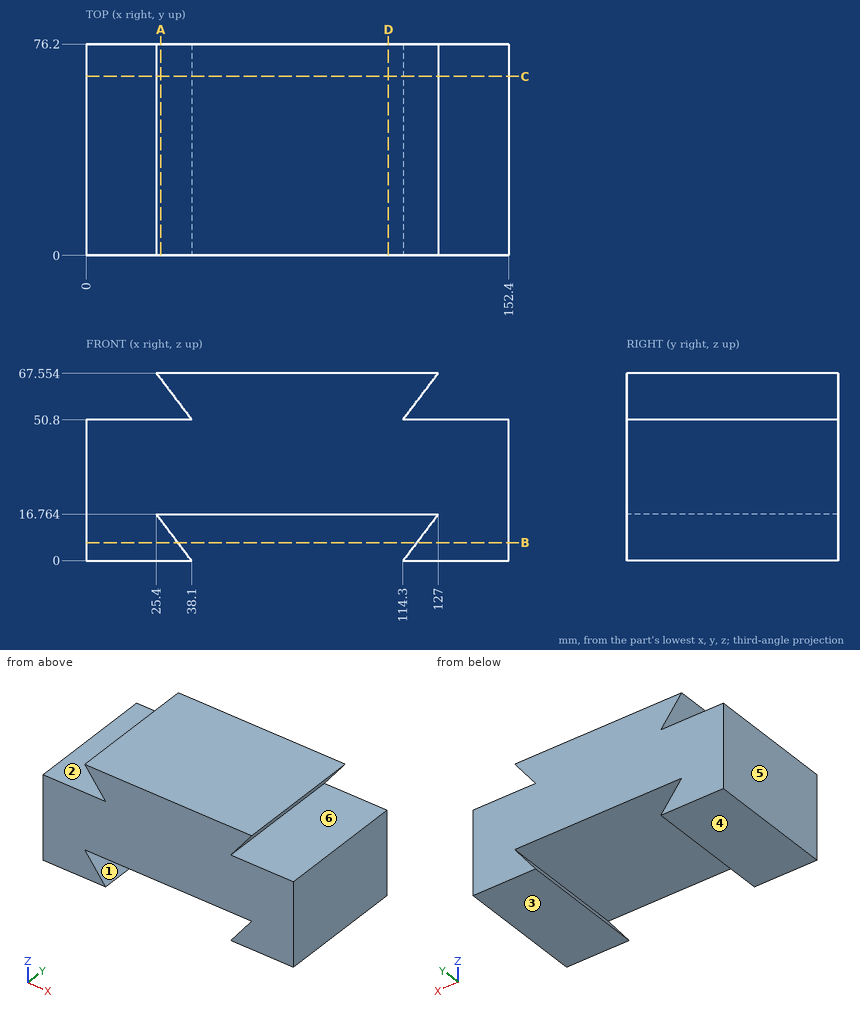
Here's the drawing with two shaded views (mm, measured from the low corner). I have some questions. A direction names the side the tool comes from. Give positions to 0.01 mm unless a question says otherwise; leave off trailing zeros. Order: outer loops, then holes, each group sorted by start corner. A loop starts at its lowest first (then second) coordinate and runs counter-clockwise, first axis right, second up. Notation, with made-up numbers: M 11.5,41 L 47.5,41 A16 cw 47.5,60 Z; hole C 5,21.5 d5. An arc over 180 degrees is marked long. One line per item, written item: value.
1) We'd pull the mould along Z, two halves only. Please class the marked faces 4, 5 and 6: released by +Z, released by -Z, zero draft, split by the parting line, or undercut.
Answer sheet:
face 4: released by -Z
face 5: zero draft
face 6: undercut
2) Please list where these lines run through material, in increasing order: line 1 along Z through (x, y) = (61, 50); line 2 along Z through (x, y) = (25, 24); line 3 along X through (y, z) = (29.5, 14) (1 decimal).
Answer sheet:
line 1: z = 16.76 to 67.55
line 2: z = 0 to 50.8
line 3: x = 0 to 27.5, 124.9 to 152.4
3) I want a section at B-B, the plane z = 6.5. List the corners of the cut face in (x, y) for me (1 decimal).
Answer sheet:
outline: M 0,0 L 33.2,0 L 33.2,76.2 L 0,76.2 Z; M 119.2,0 L 152.4,0 L 152.4,76.2 L 119.2,76.2 Z
4) For P1, Ø5, axis at x = 113.5, z = 15, coming from the -Y side; P2, Ø4, axis at x = 92, y = 27.5, coming from the -Z side, each with a flat end and sliding along its axis, tell me the tip position at first contact or that it passes through.
Answer sheet:
P1: stops at y = 0
P2: stops at z = 16.76
5) I want a section at D-D, the plane x = 109. List the corners of the cut face in (y, z) for me.
Answer sheet:
outline: M 0,16.76 L 76.2,16.76 L 76.2,67.55 L 0,67.55 Z
6) I want a section at A-A, the plane x = 27. List the corners of the cut face in (y, z) for me, plus the area to 3 significant figures.
Answer sheet:
outline: M 0,0 L 76.2,0 L 76.2,14.65 L 0,14.65 Z; M 0,16.76 L 76.2,16.76 L 76.2,50.8 L 0,50.8 Z; M 0,65.44 L 76.2,65.44 L 76.2,67.55 L 0,67.55 Z
area: 3,870 mm^2
7) I want a section at C-C, the plane y = 64.5. List the corners of the cut face in (x, z) for me, plus the area to 3 significant figures.
Answer sheet:
outline: M 0,0 L 38.1,0 L 25.4,16.76 L 127,16.76 L 114.3,0 L 152.4,0 L 152.4,50.8 L 114.3,50.8 L 127,67.55 L 25.4,67.55 L 38.1,50.8 L 0,50.8 Z
area: 7,740 mm^2
8) On a 3-axis mill with a long thin cutter (end or side, diameter ignored), from which of +Z, -Z, +X, -X, +Y, -Y can I reach the whole of each face in a straight line? I mean the marked faces 1, 2 and 3. Say none if no direction works.
Answer sheet:
face 1: +Y, -Y
face 2: -X, +Y, -Y
face 3: -Z, +X, -X, +Y, -Y
